Autodesk Inventor part; units mm, degrees
ref_plane "YZ Plane" through (0, 0, 0) normal (1, 0, 0) x (0, 1, 0)
ref_plane "XZ Plane" through (0, 0, 0) normal (0, 1, 0) x (-1, 0, 0)
ref_plane "XY Plane" through (0, 0, 0) normal (0, 0, 1) x (1, 0, 0)
sketch "Sketch1" plane through (0, 0, 0) normal (0, 0, 1) x (1, 0, 0)
  line L0 (0, 0) -> (-50.8, 0)
  line L1 (-50.8, 0) -> (-50.8, 25.4)
  line L2 (-50.8, 25.4) -> (-50.8, 76.2)
  line L3 (-50.8, 76.2) -> (0, 76.2)
  line L4 (0, 76.2) -> (0, 0)
  circle A0 centre (-38.1, 12.7) radius 3.3734
  circle A1 centre (-12.7, 38.1) radius 3.3734
  circle A2 centre (-12.7, 63.5) radius 3.3734
  circle A3 centre (-38.1, 63.5) radius 3.3734
  dimension "d0" = 50.8
  dimension "d1" = 25.4
  dimension "d2" = 76.2
  dimension "d3" = 50.8
  dimension "d4" = 6.7469
  dimension "d5" = 38.1
  dimension "d6" = 12.7
  dimension "d7" = 38.1
  dimension "d9" = 12.7
  dimension "d10" = 12.7
  dimension "d14" = 12.7
  dimension "d15" = 12.7
  dimension "d18" = 12.7
extrude "Extrusion2" add sketch "Sketch1" along normal blind 3.175
properties part number "fly wheel gusset" material "Aluminum 6061"
Work out the finished part from the listing and answer in its coordinate system (mm). Give positions to 0.01 mm unless a question says otherwise; leave off trailing zeros. Write each loop counter-clockwise with the first axis right and the second up, starting at its lowest first coordinate (ties: lowest second). Pieces come first, ordered by that corner, then holes.
(1) Straight lines are drawn through the part: line 1 (Y direction, x = -12.7, z = 1.9); line 2 (Y direction, x = -38.1, z = 1.7); line 3 (X direction, y = 66, z = 1.55). For each, find the intervals that lie inside material, in ascending order.
Final values:
line 1: y = 0 to 34.73, 41.47 to 60.13, 66.87 to 76.2
line 2: y = 0 to 9.33, 16.07 to 60.13, 66.87 to 76.2
line 3: x = -50.8 to -40.36, -35.84 to -14.96, -10.44 to 0
(2) The part is cut by section D-D on y = 63.5. Write down the section's boundary in (x, z) (3 decimals).
Final values:
outline: (-50.8, 0) - (-41.473, 0) - (-41.473, 3.175) - (-50.8, 3.175) - close; (-34.727, 0) - (-16.073, 0) - (-16.073, 3.175) - (-34.727, 3.175) - close; (-9.327, 0) - (0, 0) - (0, 3.175) - (-9.327, 3.175) - close
(3) The part is cut by section B-B on z = 1.75. Write down the section's boundary in (x, y).
Final values:
outline: (-50.8, 0) - (0, 0) - (0, 76.2) - (-50.8, 76.2) - close; hole circle Ø6.75 at (-38.1, 12.7); hole circle Ø6.75 at (-38.1, 63.5); hole circle Ø6.75 at (-12.7, 38.1); hole circle Ø6.75 at (-12.7, 63.5)
(4) The mould has two halves that part along Y. Classify faces 1 (the cylindrical face through (-13.139, 60.155, 1.565)), 2 (the cylindrical face through (-34.984, 13.992, 1.565)), 3 (the flat face through (-25, 0, 2)), 4 (the flat face through (-26, 76.2, 2)): pulls with the +Y half, pulls with the -Y half, needs draft (parallel to the pull), parting line crosses it, or undercut.
Final values:
face 1: undercut
face 2: undercut
face 3: pulls with the -Y half
face 4: pulls with the +Y half
(5) The part is cut by section A-A on y = 38.1. Write down the section's boundary in (x, z) (3 decimals), plus the area to 3 significant figures.
Final values:
outline: (-50.8, 0) - (-16.073, 0) - (-16.073, 3.175) - (-50.8, 3.175) - close; (-9.327, 0) - (0, 0) - (0, 3.175) - (-9.327, 3.175) - close
area: 140 mm2
(6) The part is cut by section C-C on x = -12.7. Write down the section's boundary in (y, z) (3 decimals), plus the area to 3 significant figures.
Final values:
outline: (0, 0) - (34.727, 0) - (34.727, 3.175) - (0, 3.175) - close; (41.473, 0) - (60.127, 0) - (60.127, 3.175) - (41.473, 3.175) - close; (66.873, 0) - (76.2, 0) - (76.2, 3.175) - (66.873, 3.175) - close
area: 199 mm2
